For this review, use the dimensioned drawing (mm, ordinates from the lowest corner) and the shaded views. Give positions to 0.01 mm unless a question says otherwise; leave off trailing zeros. Loops run counter-clockwise (first coordinate to the right, second up) from the corner with the lowest first, then second, coordinate; pieces in that order, holes last. Notation, with made-up numbers: M -28.5,72 L -4.5,72 A26 cw -4.5,110 Z; hole C -8,-13 d7. An arc over 180 degrees is marked long. Return JSON: item names as keys, results as strings.
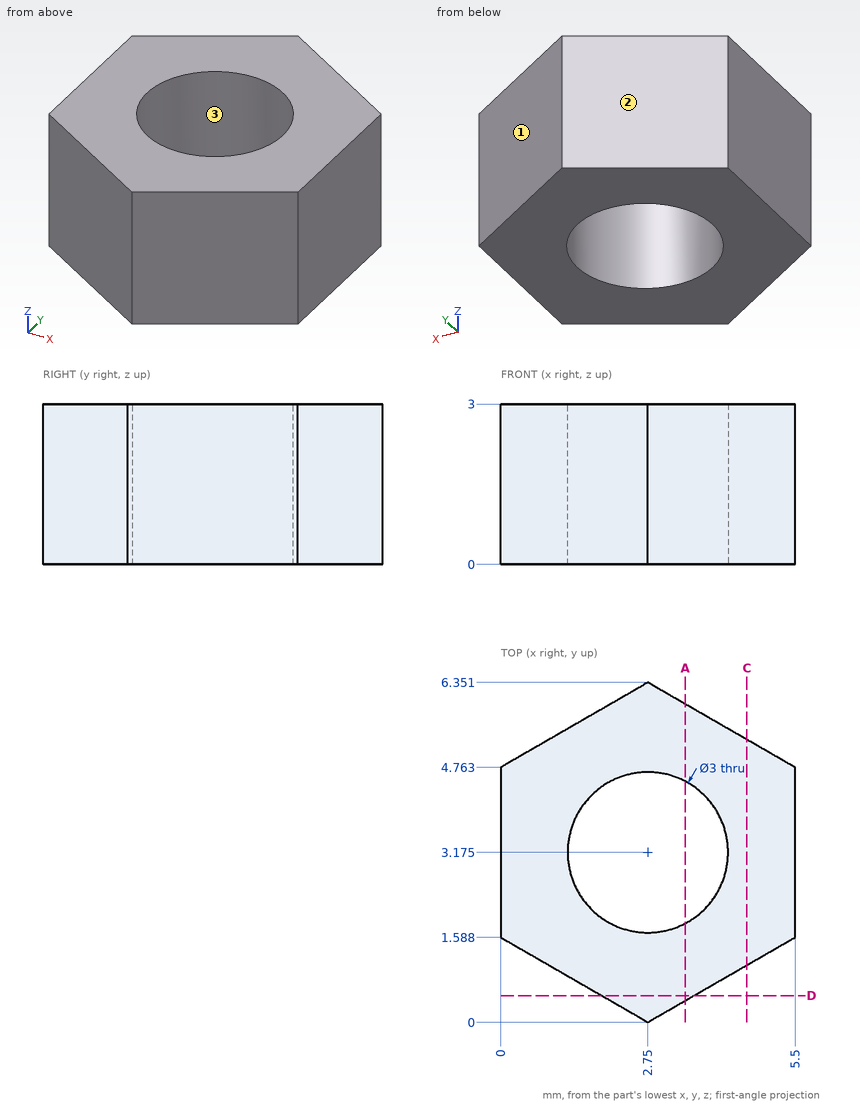
1) Consider section C-C on x = 4.6. Write out the cut boundary in (y, z).
From the geometry:
{"outline": "M 1.07,0 L 5.28,0 L 5.28,3 L 1.07,3 Z"}
2) The part is to be moulded in two halves that separate along X. For the marked faces 1, 2 and 3, say which applies: released by +X, released by -X, zero draft, split by the parting line, or undercut.
From the geometry:
{"face 1": "released by +X", "face 2": "released by -X", "face 3": "undercut"}
3) Consider section D-D on y = 0.5. Write out the cut boundary in (x, z).
From the geometry:
{"outline": "M 1.88,0 L 3.62,0 L 3.62,3 L 1.88,3 Z"}
4) Wall thickness on L1, parallel to Y at x = 1.6, z = 1.35 (1 decimal); L2, parallel to X at y = 4.25, z = 2.8 (1 decimal); L3, parallel to Y at x = 2.9, z = 0.8 (1 decimal): over which ranges is each line inside the solid? List them lowest first. Write a range as from..to.
From the geometry:
{"L1": "0.7..2.2, 4.1..5.7", "L2": "0..1.7, 3.8..5.5", "L3": "0.1..1.7, 4.7..6.3"}
5) Consider section A-A on x = 3.45. Write out the cut boundary in (y, z) (1 decimal).
From the geometry:
{"outline": "M 0.4,0 L 1.8,0 L 1.8,3 L 0.4,3 Z; M 4.5,0 L 5.9,0 L 5.9,3 L 4.5,3 Z"}
6) Insertion check: pin 1 (2 mm diameter, centred on x = 3.5, y = 1.5, fed in from -Z). The pin has a flat end and moves straight along its axis. Give the tip position at first contact, or say it passes through.
From the geometry:
{"pin 1": "z = 0"}
